Job drawing, mm, ordinate dimensions from the low corner. One solid piece. A direction names the side the tool comes from. Give positions to 0.01 mm unless a question says otherwise; leave off trailing zeros. Order: outer loops, then holes, each group sorted by start corner. A loop starts at its lowest first (then second) coordinate and runs counter-clockwise, first axis right, second up.
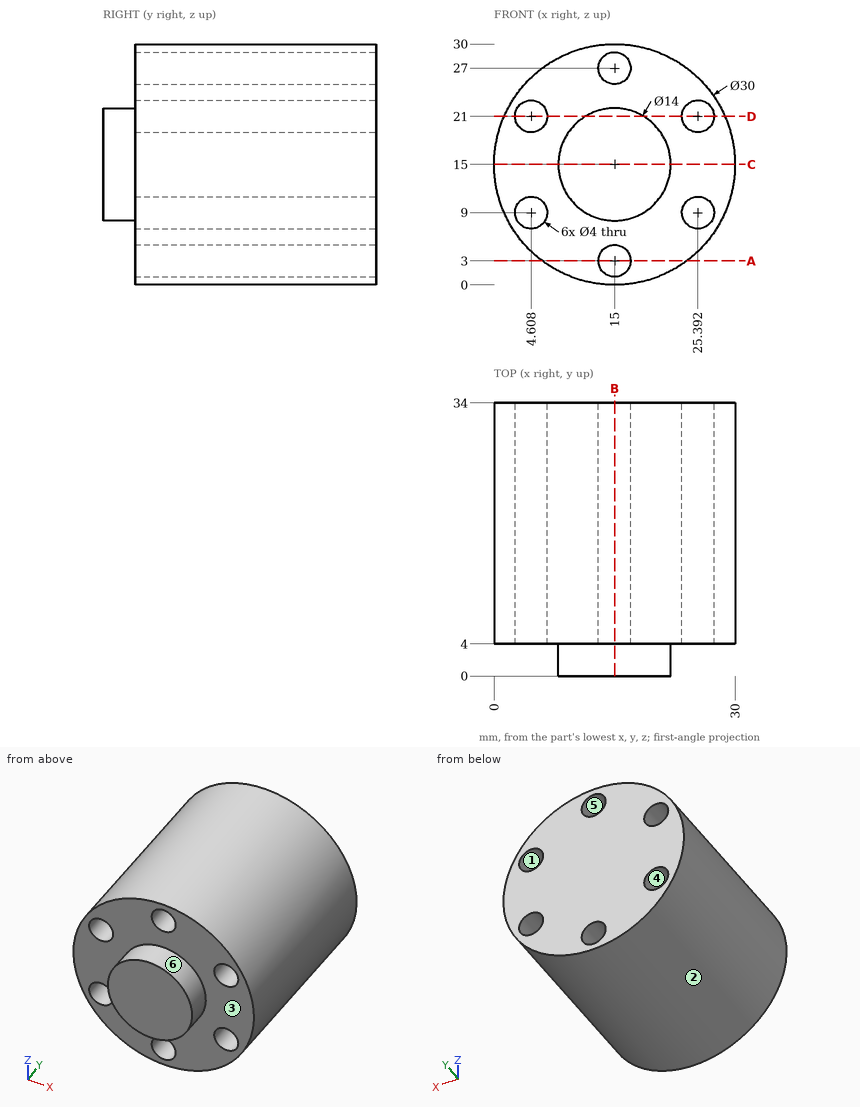
Item 1: Pull direction X, two halves, no side cores. Call the marked faces 1, 2, 3 and 4: released by +X, released by -X, zero draft, split by the parting line, or undercut.
Item 2: Band-saw the part on A-A on z = 3. List the corners of the cut face in (x, y), plus the area to 3 significant figures.
Item 3: Band-saw the part on D-D on z = 21. List the corners of the cut face in (x, y) (1 decimal).
Item 4: Band-saw the part on B-B on x = 15. List the corners of the cut face in (y, z), plus the area to 3 significant figures.
Item 5: Drop flat-ended pins along their axis: P1, Ø1, axis at x = 19.5, y = 26, coming from the -Z side; P2, Ø6, axis at x = 25, y = 15, coming from the +Z side; P3, Ø3.5, axis at x = 4.61, z = 21, coming from the +Y side; P4, Ø3, axis at y = 15.5, z = 3.5, coming from the +X side. Give the stop position or say it passes through.
Item 6: Band-saw the part on C-C on z = 15. List the corners of the cut face in (x, y).
Item 7: Drill centre lines: probe 1 along Z at (x, y) = (6, 15) (1 decimal); probe 2 along Z at (x, y) = (15.75, 18) (1 decimal); probe 3 along Y at (x, z) = (3.75, 18.5). Where is each one in solid material? Low to high.
Item 8: Which spindle directions (+Z, -Z, +X, -X, +Y, -Y) get a long thin tool onto all of the face, cutting with end or side? Do the marked faces 5 and 6. Say none if no direction does.
Working result:
1. face 1: undercut
1. face 2: split by the parting line
1. face 3: zero draft
1. face 4: undercut
2. outline: (6, 4) - (13, 4) - (13, 34) - (6, 34) - close; (17, 4) - (24, 4) - (24, 34) - (17, 34) - close
2. area: 420 mm2
3. outline: (1.3, 4) - (2.6, 4) - (2.6, 34) - (1.3, 34) - close; (6.6, 4) - (11.4, 4) - (11.4, 0) - (18.6, 0) - (18.6, 4) - (23.4, 4) - (23.4, 34) - (6.6, 34) - close; (27.4, 4) - (28.7, 4) - (28.7, 34) - (27.4, 34) - close
4. outline: (0, 8) - (4, 8) - (4, 5) - (34, 5) - (34, 25) - (4, 25) - (4, 22) - (0, 22) - close; (4, 0) - (34, 0) - (34, 1) - (4, 1) - close; (4, 29) - (34, 29) - (34, 30) - (4, 30) - close
4. area: 716 mm2
5. P1: stops at z = 0.54
5. P2: stops at z = 28.27
5. P3: passes through
5. P4: stops at x = 26.18
6. outline: (0, 4) - (8, 4) - (8, 0) - (22, 0) - (22, 4) - (30, 4) - (30, 34) - (0, 34) - close
7. probe 1: z = 3 to 7.6, 10.4 to 19.6, 22.4 to 27
7. probe 2: z = 0 to 1.1, 4.9 to 25.1, 28.9 to 30
7. probe 3: y = 4 to 34
8. face 5: +Y, -Y
8. face 6: -Y
